Could you check a few things on this model? Use its own coordinates, in mm. A direction names the side the tool comes from. Round coordinates to 2 decimals unless told otherwise and drop trailing zeros. Loops run counter-clockwise (first coordinate to the right, second up) from the corner with the lowest first, then second, coordinate; pieces in that order, holes last. Notation, with made-up numbers: (17, 75.5) -> (53, 75.5) arc R16 cw to (53, 100.5) -> close; hole circle Ø1 at (47.5, 12). An arc over 180 degrees is marked (long way). Write each question's results on one line, items separated by ' | '.
from build123d import *

# Parameters (mm, degrees)
EXTRUDE_THIN1_DEPTH = 600
FILLET2_R           = 40


with BuildPart() as part:
    # Sketch1 → Extrude-Thin1 (new body)
    with BuildSketch(Plane.XY):
        Polygon((-32.139380484, -38.302222156), (0, 0), (70, 0), (95.711504387, -30.641777725), (103.371948819, -24.213901628), (74.663076582, 10), (-4.663076582, 10), (-39.799824916, -31.874346059), align=None)
    extrude(amount=EXTRUDE_THIN1_DEPTH)

    # Fillet2
    # the kernel refuses this fillet: 40 mm, written as the material it takes off along each edge
    with BuildSketch(Plane(origin=(74.663076582, 10, -46.630765815), x_dir=(0.6427876096865376, -0.7660444431189795, 0), z_dir=(0, 0, 1)), Plane(origin=(-4.663076582, 10, -46.630765815), x_dir=(1, 0, 0), z_dir=(0, 0, 1))) as fillet2_piece_1:
        with BuildLine():
            CenterArc((FILLET2_R * 0.466307658155, -FILLET2_R), FILLET2_R, 90, 50)
            Line((-FILLET2_R * 0.299736784964, -FILLET2_R * 0.357212390313), (0, 0))
            Line((0, 0), (FILLET2_R * 0.466307658155, 0))
        make_face()
    extrude(amount=693.261531631, mode=Mode.SUBTRACT)
    with BuildSketch(Plane(origin=(174.663076582, 10, 600), x_dir=(0, 0, -1), z_dir=(-1, 0, 0))) as fillet2_piece_2:
        with BuildLine():
            CenterArc((FILLET2_R, FILLET2_R), FILLET2_R, 180, 90)
            Line((0, FILLET2_R), (0, 0))
            Line((0, 0), (FILLET2_R, 0))
        make_face()
    extrude(amount=279.326153163, mode=Mode.SUBTRACT)
    with BuildSketch(Plane(origin=(174.663076582, 10, 0), x_dir=(0, 0, 1), z_dir=(-1, 0, 0))) as fillet2_piece_3:
        with BuildLine():
            CenterArc((FILLET2_R, -FILLET2_R), FILLET2_R, 90, 90)
            Line((0, -FILLET2_R), (0, 0))
            Line((0, 0), (FILLET2_R, 0))
        make_face()
    extrude(amount=279.326153163, mode=Mode.SUBTRACT)


solid = part.part
1) For faces 4 (the flat face through (-16.295, -19.419, 295.8)), 5 (the cylindrical face through (73.137, 6.148, 295.931)), which set-ups out of +Z, -Z, +X, -X, +Y, -Y let a thin tool reach every point of the face, with its end or its side?
Model answer:
face 4: +Z, -Z, -Y | face 5: +Z, -Z, +X, +Y
2) I need wall thicknesses on line 1 (X direction, y = -30, z = 83); line 2 (Y direction, x = 15.5, z = 258); line 3 (Y direction, x = 7.5, z = 91). Which ranges of each line are inside material? Lowest first, please.
Model answer:
line 1: x = -38.23 to -25.17, 95.17 to 96.48 | line 2: y = 0 to 10 | line 3: y = 0 to 9.47
3) I want a section at A-A, the plane z = 332. Write out the boundary of the cut face in (x, y).
Model answer:
outline: (-39.8, -31.87) -> (-32.14, -38.3) -> (0, 0) -> (70, 0) -> (95.71, -30.64) -> (103.37, -24.21) -> (86.65, -4.29) arc R40 ccw to (56.01, 10) -> (13.99, 10) arc R40 ccw to (-16.65, -4.29) -> close
4) I want a section at C-C, the plane x = 44. Write out the boundary of the cut face in (y, z), plus the area to 3 significant figures.
Model answer:
outline: (0, 13.54) arc R40 ccw to (10, 40) -> (10, 560) arc R40 ccw to (0, 586.46) -> close | area: 5,560 mm2
5) I'm going to push flat-ended pins straight in: pin 1 (6 mm diameter, centred on y = -12.5, z = 179, fed in from +X); pin 2 (12 mm diameter, centred on x = 5, y = 4.5, fed in from -Z); pin 3 (12 mm diameter, centred on x = 73.5, y = -1, fed in from -Z). Where does each tip first touch, or does it pass through?
Model answer:
pin 1: stops at x = 96.06 | pin 2: stops at z = 13.54 | pin 3: stops at z = 7.53
6) If we mould it in two halves opening along X, with no side actions, what happens to faces 1 (the flat face through (95.13, -14.39, 295.81)), 2 (the flat face through (82.68, -15.11, 295.8)), 3 (the cylindrical face through (-2.694, 6.355, 295.931))? For each: released by +X, released by -X, zero draft, split by the parting line, or undercut.
Model answer:
face 1: released by +X | face 2: undercut | face 3: released by -X
7) I want a section at B-B, the plane y = -19. Write out the boundary of the cut face in (x, z), plus the area to 3 significant figures.
Model answer:
outline: (-29, 1.54) -> (-15.94, 1.54) -> (-15.94, 598.46) -> (-29, 598.46) -> close; (85.94, 1.54) -> (99, 1.54) -> (99, 598.46) -> (85.94, 598.46) -> close | area: 15,600 mm2
8) I want a section at D-D, the plane y = 5. Write out the boundary of the cut face in (x, z), plus the area to 3 significant figures.
Model answer:
outline: (-5.38, 20.64) -> (75.38, 20.64) -> (75.38, 579.36) -> (-5.38, 579.36) -> close | area: 45,100 mm2
